For this review, take the finished solid that the model builds, in its own axes (mm). A direction names the side the tool comes from. Coordinates: 2 decimals unless noted, no trailing zeros. Write each loop counter-clockwise with the first axis right and the second up, starting at its lowest first coordinate (ties: lowest second). Pieces come first, ordered by that corner, then holes. Notation, with made-up numbers: M 45,33.25 L 53,33.25 A17 ccw 53,37.25 Z; hole C 71,70.25 d10. An arc over 180 degrees is marked long. One line per question, with ' | ' between items.
from build123d import *

# Parameters (mm, degrees)
SKETCH1_R               = 12
BOSS_EXTRUDE1_DEPTH     = 24
BOSS_EXTRUDE2_START     = 12
SKETCH1_4_R             = 18
SKETCH1_4_R_2           = 14.5
SKETCH1_4_R_3           = 12
BOSS_EXTRUDE2_DEPTH     = 12
BOSS_EXTRUDE4_START     = 12
SKETCH1_8_R             = 14.5
BOSS_EXTRUDE4_DEPTH     = 70
CUT_EXTRUDE1_DEPTH      = 86.860351735
CUT_EXTRUDE1_DEPTH_BACK = 86.860351735
SKETCH2_W               = 8
SKETCH2_H               = 34


with BuildPart() as part:
    # Sketch1 → Boss-Extrude1 (new body)
    with BuildSketch(Plane(origin=(0, 0, 0), x_dir=(1, 0, 0), z_dir=(0, 1, 0))):
        with Locations(Location((0, 0, 0), (0, 0, 270))):
            Circle(SKETCH1_R)
    extrude(amount=-BOSS_EXTRUDE1_DEPTH)

    # Sketch1<4> → Boss-Extrude2 (add)
    # profile 1 of 3: a face of its own
    with BuildSketch(Plane(origin=(0, 0, 0), x_dir=(1, 0, 0), z_dir=(0, 1, 0)).offset(BOSS_EXTRUDE2_START)):
        with Locations(Location((0, 0, 0), (0, 0, 270))):
            Circle(SKETCH1_4_R)
        Circle(SKETCH1_4_R_2, mode=Mode.SUBTRACT)
    # profile 2 of 3: a face of its own
    with BuildSketch(Plane(origin=(0, 0, 0), x_dir=(1, 0, 0), z_dir=(0, 1, 0)).offset(BOSS_EXTRUDE2_START)):
        Circle(SKETCH1_4_R_2)
        with Locations(Location((0, 0, 0), (0, 0, 270))):
            Circle(SKETCH1_4_R_3, mode=Mode.SUBTRACT)
    # profile 3 of 3: a face of its own
    with BuildSketch(Plane(origin=(0, 0, 0), x_dir=(1, 0, 0), z_dir=(0, 1, 0)).offset(BOSS_EXTRUDE2_START)):
        with Locations(Location((0, 0, 0), (0, 0, 270))):
            Circle(SKETCH1_4_R_3)
    extrude(amount=-BOSS_EXTRUDE2_DEPTH)

    # Sketch1<8> → Boss-Extrude4 (add)
    with BuildSketch(Plane(origin=(0, 0, 0), x_dir=(1, 0, 0), z_dir=(0, 1, 0)).offset(BOSS_EXTRUDE4_START)):
        with Locations(Location((0, 0, 0), (0, 0, 270))):
            Circle(SKETCH1_8_R)
    extrude(amount=BOSS_EXTRUDE4_DEPTH)

    # Sketch2 → Cut-Extrude1 (cut, two sides: drawn at the far end of the back side and taken through both)
    with BuildSketch(Plane.XY.offset(-CUT_EXTRUDE1_DEPTH_BACK)):
        with Locations((0, 47)):
            Rectangle(SKETCH2_W, SKETCH2_H)
    extrude(amount=CUT_EXTRUDE1_DEPTH + CUT_EXTRUDE1_DEPTH_BACK, mode=Mode.SUBTRACT)


solid = part.part
1) We need section B-B on x = 0. State the section outline as (y, z) points.
Responses:
outline: M -24,-12 L 0,-12 L 0,-18 L 12,-18 L 12,-14.5 L 30,-14.5 L 30,14.5 L 12,14.5 L 12,18 L 0,18 L 0,12 L -24,12 Z; M 64,-14.5 L 82,-14.5 L 82,14.5 L 64,14.5 Z
2) To check wall thickness, follow line 1 along Y through (x, z) = (-2, 4.5); line 2 along Y through (x, z) = (-12, 9.5); line 3 along X through (y, z) = (46.5, -9). State the ranges of each line that lie inside material, in increasing order. Write a range as [from, to].
Responses:
line 1: [-24, 30], [64, 82] | line 2: [0, 12] | line 3: [-11.37, -4], [4, 11.37]
3) Insertion check: pin 1 Ø8.5 at (y, z) = (53.5, -6) entering from +X; pin 2 Ø1.5 at (x, y) = (10.5, 43.5) entering from -Z; pin 3 Ø5 at (y, z) = (50.5, -10.5) entering from +X. Each pin has a flat end and moves straight along its axis. Give the tip position at first contact, or say it passes through.
Responses:
pin 1: x = 14.39 | pin 2: z = -10.73 | pin 3: x = 12.09
4) We need section C-C on y = -6. State the section outline as (x, z) points, then the cut area to 3 significant figures.
Responses:
outline: C 0,0 d24 | area: 452 mm^2
5) We need section A-A on z = 0. State the section outline as (x, y) points.
Responses:
outline: M -18,0 L -12,0 L -12,-24 L 12,-24 L 12,0 L 18,0 L 18,12 L 14.5,12 L 14.5,82 L -14.5,82 L -14.5,12 L -18,12 Z; hole M -4,30 L 4,30 L 4,64 L -4,64 Z
6) The part is to be moulded in two halves that separate along Y. For faces 1 (the flat face through (4, 47, 0)), 2 (the flat face through (-4, 47, 0)), 3 (the flat face through (-12, 0, 4)), 4 (the flat face through (0, 82, 0)), say which applies: +Y half, -Y half, draft (parallel to the pull), parting line (faces both ways), or undercut.
Responses:
face 1: undercut | face 2: undercut | face 3: -Y half | face 4: +Y half
7) Machinability: for faces 5 (the cylindrical face through (-5.554, 46.51, 13.394)), 6 (the cylindrical face through (3.604, -11.832, 11.446)), 7 (the flat face through (0, 30, 0)), 8 (the cylindrical face through (5.407, 6.084, 17.169)), 9 (the flat face through (0, -24, 0)), which of the approach directions +Z, -Z, +X, -X, +Y, -Y give a long, thin tool a straight path to every point of the face, cutting with its end or side? Answer none if there is none.
Responses:
face 5: +Y | face 6: -Y | face 7: +Z, -Z | face 8: +Y, -Y | face 9: +Z, -Z, +X, -X, -Y
8) We need section D-D on x = -11. State the section outline as (y, z) points, then the cut area to 3 significant figures.
Responses:
outline: M -24,-4.8 L 0,-4.8 L 0,-14.25 L 12,-14.25 L 12,-9.45 L 82,-9.45 L 82,9.45 L 12,9.45 L 12,14.25 L 0,14.25 L 0,4.8 L -24,4.8 Z | area: 1,890 mm^2
